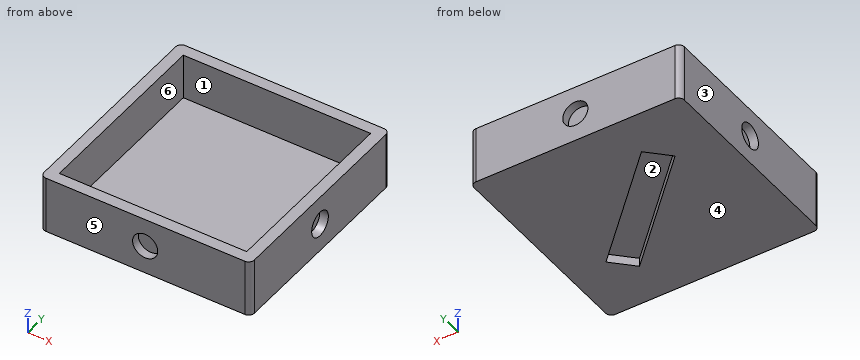
from build123d import *

# Parameters (mm, degrees)
F0_W        = 65.5
F0_H        = 65.5
F1_DEPTH    = 16
F2_T        = 4
F3_T1_DEPTH = 30
F4_R        = 4.4
F8_DEPTH    = 3
F9_DEPTH    = 3
F5_R        = 4.4
F10_DEPTH   = 3
F6_R        = 4.4
F11_DEPTH   = 3
F7_R        = 4.4
F12_DEPTH   = 3
F14_DEPTH   = 3


# Not quite as in the source:
# - a fillet or chamfer that OpenCascade refuses, or shapes differently, is made with other operations: its cross-section is extruded or revolved along the edge and cut away or added


with BuildPart() as f1:
    # F0 (on Top) → F1 (new body)
    with BuildSketch(Plane.XY):
        with Locations((4.3041806072, -3.8802318871)):
            Rectangle(F0_W, F0_H)
    extrude(amount=F1_DEPTH)

    # F2
    f2_openings = [f1.faces().sort_by_distance(p)[0] for p in [
        (4.304181, -3.880232, 16),
    ]]
    offset(amount=F2_T, openings=f2_openings, kind=Kind.INTERSECTION)

    # F3: fillet of radius 2 on 4 edges, made by hand

    # F3_s2 → F3_t1 (cut)
    with BuildSketch(Plane.XY.offset(-9)):
        with BuildLine():
            ThreePointArc((41.0541806072, -38.6302318871), (40.4683941696, -40.0444454495), (39.0541806072, -40.6302318871))
            Line((39.0541806072, -40.6302318871), (41.0541806072, -40.6302318871))
            Line((41.0541806072, -40.6302318871), (41.0541806072, -38.6302318871))
        make_face()
        with BuildLine():
            ThreePointArc((41.0541806072, 30.8697681129), (40.4683941696, 32.2839816753), (39.0541806072, 32.8697681129))
            Line((39.0541806072, 32.8697681129), (41.0541806072, 32.8697681129))
            Line((41.0541806072, 32.8697681129), (41.0541806072, 30.8697681129))
        make_face()
        with BuildLine():
            ThreePointArc((-30.4458193928, 32.8697681129), (-31.8600329552, 32.2839816753), (-32.4458193928, 30.8697681129))
            Line((-32.4458193928, 30.8697681129), (-32.4458193928, 32.8697681129))
            Line((-32.4458193928, 32.8697681129), (-30.4458193928, 32.8697681129))
        make_face()
        with BuildLine():
            ThreePointArc((-32.4458193928, -38.6302318871), (-31.8600329552, -40.0444454495), (-30.4458193928, -40.6302318871))
            Line((-30.4458193928, -40.6302318871), (-32.4458193928, -40.6302318871))
            Line((-32.4458193928, -40.6302318871), (-32.4458193928, -38.6302318871))
        make_face()
    extrude(amount=F3_T1_DEPTH, mode=Mode.SUBTRACT)

    # F4 (on face) → F8 (join)
    with BuildSketch(Plane(origin=(-32.4458193928, 0, 0), x_dir=(0, -1, 0), z_dir=(-1, 0, 0))):
        with Locations((3.8802318871, 6)):
            Circle(F4_R)
    extrude(amount=-F8_DEPTH)

    # F4 (on face) → F9 (cut)
    with BuildSketch(Plane(origin=(-32.4458193928, 0, 0), x_dir=(0, -1, 0), z_dir=(-1, 0, 0))):
        with Locations((3.8802318871, 6)):
            Circle(F4_R)
    extrude(amount=-F9_DEPTH, mode=Mode.SUBTRACT)

    # F5 (on face) → F10 (cut)
    with BuildSketch(Plane.XZ.offset(40.6302318871)):
        with Locations((4.2000180173, 6.0547004089)):
            Circle(F5_R)
    extrude(amount=-F10_DEPTH, mode=Mode.SUBTRACT)

    # F6 (on face) → F11 (cut)
    with BuildSketch(Plane.YZ.offset(41.0541806072)):
        with Locations((-3.9293510383, 6.0207889489)):
            Circle(F6_R)
    extrude(amount=-F11_DEPTH, mode=Mode.SUBTRACT)

    # F7 (on face) → F12 (cut)
    with BuildSketch(Plane(origin=(0, 32.8697681129, 0), x_dir=(-1, 0, 0), z_dir=(0, 1, 0))):
        with Locations((-4.345219037, 6.0662772571)):
            Circle(F7_R)
    extrude(amount=-F12_DEPTH, mode=Mode.SUBTRACT)

    # F13 (on face) → F14 (cut)
    with BuildSketch(Plane(origin=(0, 0, -4), x_dir=(1, 0, 0), z_dir=(0, 0, -1))):
        Polygon((27.9313208005, 18.9403499991), (20.8531849213, 26.0043426715), (-15.9149708404, -10.7666407574), (-8.8368349613, -17.8306334298), align=None)
    extrude(amount=-F14_DEPTH, mode=Mode.SUBTRACT)


solid = f1.part
CAD build for the part. Positions are in the model's coordinates, mm. Face numbers are marked on the shaded views. A direction names the side the tool comes from. Round coordinates to 2 decimals unless told otherwise and drop trailing zeros. Write each loop counter-clockwise with the first axis right and the second up, starting at its lowest first coordinate (ties: lowest second). Pieces come first, ordered by that corner, then holes.
(1) Slice it at D-D, the plane y = -0.5. Write the cut outline in (x, z).
(2) Drop flat-ended pins along their axis: P1, Ø4.5, axis at x = 4, z = 6, coming from the -Y side; P2, Ø3, axis at x = 14.5, y = -3.5, coming from the +Z side. Give the stop position or say it passes through.
(3) Probe line 1 along X through (y, z) = (-22.5, 10.75); line 2 along X through (y, z) = (-3.5, 7.25); line 3 along Y through (x, z) = (-20.5, 11.5). List the from-to ranges inside material, lowest first.
(4) Slice it at B-B, the plane y = 26. Write the cut outline in (x, z).
(5) Mould opens along Y. For the marked faces 4, 5 and 6 say: pulls with the +Y half, pulls with the -Y half, needs draft (parallel to the pull), parting line crosses it, or undercut.
(6) Slice it at C-C, the plane x = 12.5. Write the cut outline in (y, z).
(7) 3-axis set-ups, long thin cutter, end or side, ignore diameter. For the marked faces 1, 2 and 3: which of +Z, -Z, +X, -X, +Y, -Y reach the whole face in a straight line?
(8) Slice it at A-A, the plane z = 13.75. Write the cut outline in (x, y), and give its area (3 significant figures).
From the geometry:
1. outline: (-32.45, -4) - (-4.65, -4) - (-4.65, -1) - (9.49, -1) - (9.49, -4) - (41.05, -4) - (41.05, 3.26) - (38.05, 3.26) - (38.05, 8.78) - (41.05, 8.78) - (41.05, 16) - (37.05, 16) - (37.05, 0) - (-28.45, 0) - (-28.45, 16) - (-32.45, 16) - (-32.45, 8.82) - (-29.45, 8.82) - (-29.45, 3.18) - (-32.45, 3.18) - close
2. P1: stops at y = -37.63
2. P2: stops at z = 0
3. line 1: x = -32.45 to -28.45, 37.05 to 41.05
3. line 2: x = -29.45 to -28.45, 37.05 to 38.05
3. line 3: y = -40.63 to -36.63, 28.87 to 32.87
4. outline: (-32.45, -4) - (41.05, -4) - (41.05, 16) - (37.05, 16) - (37.05, 0) - (-28.45, 0) - (-28.45, 16) - (-32.45, 16) - close
5. face 4: needs draft
5. face 5: pulls with the -Y half
5. face 6: undercut
6. outline: (-40.63, -4) - (-17.65, -4) - (-17.65, -1) - (-3.51, -1) - (-3.51, -4) - (32.87, -4) - (32.87, 16) - (28.87, 16) - (28.87, 0) - (-36.63, 0) - (-36.63, 16) - (-40.63, 16) - close
7. face 1: +Z
7. face 2: -Z
7. face 3: +Z, -Z, -X, +Y, -Y
8. outline: (-32.45, -38.63) arc R2 ccw to (-30.45, -40.63) - (39.05, -40.63) arc R2 ccw to (41.05, -38.63) - (41.05, 30.87) arc R2 ccw to (39.05, 32.87) - (-30.45, 32.87) arc R2 ccw to (-32.45, 30.87) - close; hole (-28.45, -36.63) - (37.05, -36.63) - (37.05, 28.87) - (-28.45, 28.87) - close
8. area: 1,110 mm2
